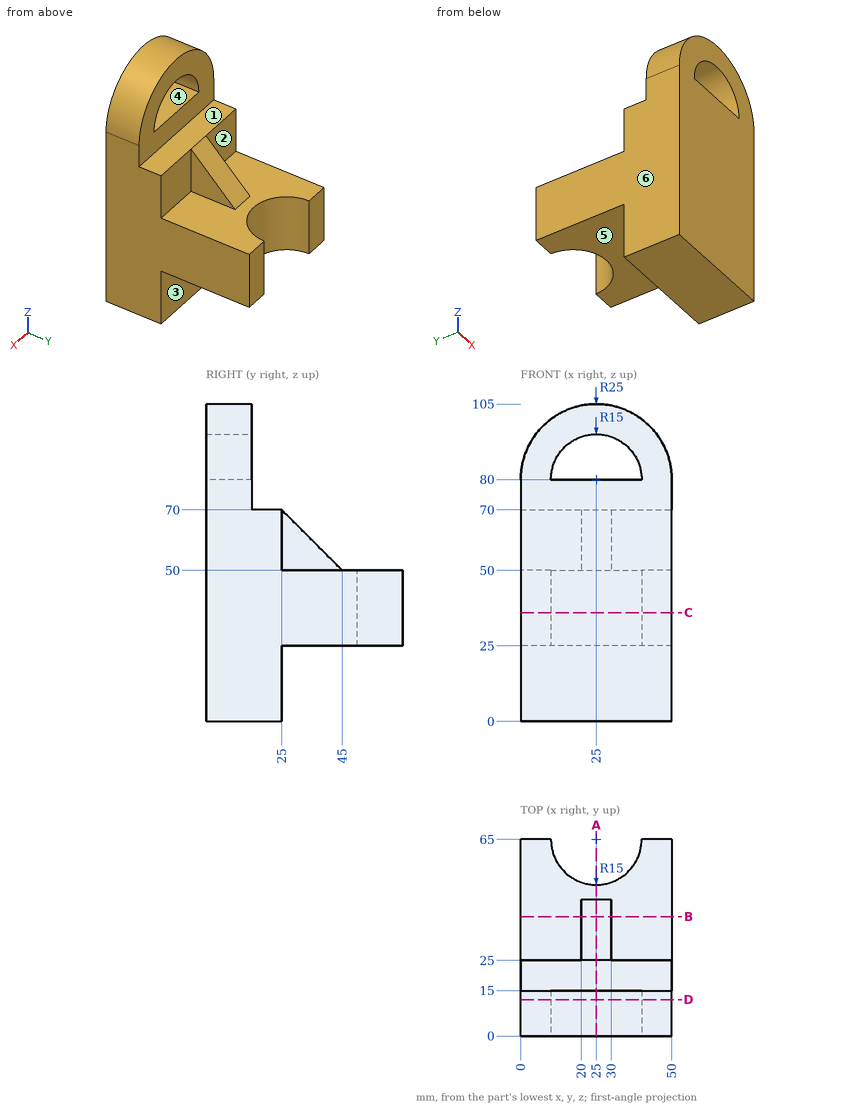
Geometry check sheet. Reference: drawing and pictorial views, mm from the part's lowest x, y, z. A direction names the side the tool comes from. Round coordinates to 2 decimals unless told otherwise and drop trailing zeros. Order: outer loops, then holes, each group sorted by start corner. A loop starts at its lowest first (then second) coordinate and runs counter-clockwise, first axis right, second up. Notation, with made-up numbers: (68.25, 61.5) - (98.25, 61.5) arc R30 ccw to (98.25, 93.5) - close; hole circle Ø9 at (82.25, 5.5). An arc over 180 degrees is marked (long way). Use a Markdown table: item, result. Add a question column.
1) Section check B-B (y = 39.5). Record the cut outline in (x, z), then the cut area to 4 significant figures.
2) Thickness scan on line 1 along Z through (x, y) = (33.5, 29); line 2 along Z through (x, y) = (36, 20); line 3 along Z through (x, y) = (35, 5). Record the ranges inside material, lowest first.
3) Mould release check, pull along X, two halves, no side actions. Record for the marked faces 4, 5 and 6: released by +X, released by -X, zero draft, split by the parting line, or undercut.
4) Section check D-D (y = 12). Record the cut outline in (x, z).
5) Section check A-A (x = 25). Record the cut outline in (y, z).
6) Set-up check for the marked faces 1, 2 and 3: record each of +Z, -Z, +X, -X, +Y, -Y from which the full face is reachable in a straight line by a thin tool's end or side.
7) Gauge pin test, flat ends, axial feed: P1, Ø4, axis at x = 14, y = 52.5, coming from the +Z side; P2, Ø22, axis at x = 15, z = 56.5, coming from the +Y side; P3, Ø16, axis at x = 43, z = 63, coming from the +Y side; P4, Ø12, axis at x = 6, y = 27.5, coming from the +Z side. Record the tip position at first contact, or that the pin passes through.
8) Section check C-C (z = 36). Record the cut outline in (x, y).
Established:
| question | item | result |
|---|---|---|
| 1 | outline | (0, 25) - (50, 25) - (50, 50) - (30, 50) - (30, 55.5) - (20, 55.5) - (20, 50) - (0, 50) - close |
| 1 | area | 1,305 mm2 |
| 2 | line 1 | 25 to 50 |
| 2 | line 2 | 0 to 70 |
| 2 | line 3 | 0 to 80, 91.18 to 102.91 |
| 3 | face 4 | undercut |
| 3 | face 5 | zero draft |
| 3 | face 6 | released by -X |
| 4 | outline | (0, 0) - (50, 0) - (50, 80) arc R25 ccw to (0, 80) - close; hole (10, 80) - (40, 80) arc R15 ccw to start |
| 5 | outline | (0, 0) - (25, 0) - (25, 25) - (50, 25) - (50, 50) - (45, 50) - (25, 70) - (15, 70) - (15, 80) - (0, 80) - close; (0, 95) - (15, 95) - (15, 105) - (0, 105) - close |
| 6 | face 1 | +Z, +X, -X, +Y |
| 6 | face 2 | +Z, -X, +Y |
| 6 | face 3 | -Z, +X, -X, +Y |
| 7 | P1 | z = 50 |
| 7 | P2 | y = 65 |
| 7 | P3 | y = 25 |
| 7 | P4 | z = 70 |
| 8 | outline | (0, 0) - (50, 0) - (50, 65) - (40, 65) arc R15 cw to (10, 65) - (0, 65) - close |
